The listing builds one solid part. Answer for the finished solid, in the listing's coordinates (mm). A direction names the side the tool comes from. Coordinates: 2 decimals unless noted, no trailing zeros. One line per question, with ' | ' between items.
from build123d import *

# Parameters (mm, degrees)
SKETCH2_W            = 20
SKETCH2_H            = 20
BOSS_EXTRUDE1_DEPTH  = 400
CUT_EXTRUDE1_DEPTH   = 401.249921924
CIRPATTERN2_COUNT    = 4
SKETCH9_R            = 2.1
CUT_EXTRUDE2_DEPTH   = 401.249921924
MIRROR1_COPY_1_DEPTH = 401.249921924
MIRROR1_COPY_2_DEPTH = 401.249921924
MIRROR1_COPY_3_DEPTH = 401.249921924
CUT_EXTRUDE3_DEPTH   = 402.248052955
FILLET1_R            = 1


with BuildPart() as part:
    # Sketch2 → Boss-Extrude1 (new body)
    with BuildSketch(Plane.XY):
        Rectangle(SKETCH2_W, SKETCH2_H)
    boss_extrude1 = extrude(amount=-BOSS_EXTRUDE1_DEPTH)

    # Sketch3 → Cut-Extrude1 (cut, symmetric)
    with BuildSketch(Plane.XY):
        Polygon((-3.1, 8.2), (-4.9, 10), (4.9, 10), (3.1, 8.2), (5.5, 8.2), (5.5, 6.56), (2.84, 3.9), (-2.84, 3.9), (-5.5, 6.56), (-5.5, 8.2), align=None)
    cut_extrude1 = extrude(amount=CUT_EXTRUDE1_DEPTH, both=True, mode=Mode.SUBTRACT)

    # CirPattern2: Cut-Extrude1 ×4 about axis
    cirpattern2_axis = Axis((0, 0, 0), (0, 0, 1))
    for i in range(1, CIRPATTERN2_COUNT):
        add(cut_extrude1.rotate(cirpattern2_axis, i * 360 / CIRPATTERN2_COUNT), mode=Mode.SUBTRACT)

    # Sketch9 → Cut-Extrude2 (cut, through all)
    with BuildSketch(Plane.XY):
        Circle(SKETCH9_R)
    cut_extrude2 = extrude(amount=-CUT_EXTRUDE2_DEPTH, mode=Mode.SUBTRACT)

    # Mirror1: Boss-Extrude1, Cut-Extrude1, Cut-Extrude2 across plane
    add(boss_extrude1.mirror(Plane(origin=(10, 10, -400), x_dir=(0, 0, 1), z_dir=(1, 0, 0))))
    add(cut_extrude1.mirror(Plane(origin=(10, 10, -400), x_dir=(0, 0, 1), z_dir=(1, 0, 0))), mode=Mode.SUBTRACT)
    add(cut_extrude2.mirror(Plane(origin=(10, 10, -400), x_dir=(0, 0, 1), z_dir=(1, 0, 0))), mode=Mode.SUBTRACT)

    # Mirror1 copy 1 sketch → Mirror1 copy 1 (cut, symmetric)
    with BuildSketch(Plane(origin=(20, 0, 0), x_dir=(0, 1, 0), z_dir=(0, 0, 1))):
        Polygon((-3.1, -8.2), (-4.9, -10), (4.9, -10), (3.1, -8.2), (5.5, -8.2), (5.5, -6.56), (2.84, -3.9), (-2.84, -3.9), (-5.5, -6.56), (-5.5, -8.2), align=None)
    extrude(amount=MIRROR1_COPY_1_DEPTH, both=True, mode=Mode.SUBTRACT)

    # Mirror1 copy 2 sketch → Mirror1 copy 2 (cut, symmetric)
    with BuildSketch(Plane(origin=(20, 0, 0), x_dir=(1, 0, 0), z_dir=(0, 0, 1))):
        Polygon((-3.1, -8.2), (-4.9, -10), (4.9, -10), (3.1, -8.2), (5.5, -8.2), (5.5, -6.56), (2.84, -3.9), (-2.84, -3.9), (-5.5, -6.56), (-5.5, -8.2), align=None)
    extrude(amount=MIRROR1_COPY_2_DEPTH, both=True, mode=Mode.SUBTRACT)

    # Mirror1 copy 3 sketch → Mirror1 copy 3 (cut, symmetric)
    with BuildSketch(Plane(origin=(20, 0, 0), x_dir=(0, -1, 0), z_dir=(0, 0, 1))):
        Polygon((-3.1, -8.2), (-4.9, -10), (4.9, -10), (3.1, -8.2), (5.5, -8.2), (5.5, -6.56), (2.84, -3.9), (-2.84, -3.9), (-5.5, -6.56), (-5.5, -8.2), align=None)
    extrude(amount=MIRROR1_COPY_3_DEPTH, both=True, mode=Mode.SUBTRACT)

    # Sketch10 → Cut-Extrude3 (cut, through all)
    with BuildSketch(Plane.XY):
        Polygon((13.44, -5.5), (11.8, -5.5), (8.2, -5.5), (6.56, -5.5), (6.56, 5.5), (8.2, 5.5), (11.8, 5.5), (13.44, 5.5), align=None)
    extrude(amount=-CUT_EXTRUDE3_DEPTH, mode=Mode.SUBTRACT)

    # Fillet1
    fillet1_edges = [part.edges().sort_by_distance(p)[0] for p in [
        (30, 10, -200),
        (30, -10, -200),
        (-10, 10, -200),
        (-10, -10, -200),
    ]]
    fillet(fillet1_edges, radius=FILLET1_R)


solid = part.part
Item 1: For faces 1 (the face through (15, 5, -400)), 2 (the face through (10, -5.5, -197)), determine the directions among +Z, -Z, +X, -X, +Y, -Y from which every point of the face is accessible in a straight line to the end or side of a thin tool.
Computed values:
face 1: -Z, +X, -X, +Y, -Y | face 2: +Z, -Z
Item 2: Determine the mould class of faces 3 (the face through (15, 5, 0)), 4 (the face through (10, 10, -197)), 5 (the face through (10, 5.5, -197)) for opening direction Y: pulls with the +Y half, pulls with the -Y half, needs draft (parallel to the pull), parting line crosses it, or undercut.
Computed values:
face 3: needs draft | face 4: pulls with the +Y half | face 5: undercut
Item 3: Each of these flat-tipped pins is pushed along its axis until it touches: pin 1 Ø4.5 at (x, z) = (21.5, -286.5) entering from -Y; pin 2 Ø1.7 at (x, z) = (1.5, -286.5) entering from -Y; pin 3 Ø6 at (y, z) = (1, -171) entering from +X. Where does it stop, or does it pass through?
Computed values:
pin 1: stops at y = -8.85 | pin 2: stops at y = -3.9 | pin 3: stops at x = 29.1
Item 4: Section A-A, the plane z = -292 is taken. Count the separate pieces of the cut face and the enclosed holes in it, plus the area to 3 significant figures.
Computed values:
separate pieces: 1 | enclosed holes: 3 | area: 324 mm^2
Item 5: Find the intervals of material crossed by L1, parallel to X at y = 0.25, z = -312; L2, parallel to X at y = -7, z = -245.5; L3, parallel to Y at x = 6, z = -75, in increasing order.
Computed values:
L1: x = -3.9 to -2.09, 2.09 to 3.9, 16.1 to 17.91, 22.09 to 23.9 | L2: x = -10 to -5.5, 5.5 to 14.5, 25.5 to 30 | L3: y = -10 to -4.94, 4.94 to 10
